Answer from the drawing. Dimensions are ordinates in mm from the lowest x, y and z of the part. Coordinates: 2 decimals unless noted, no trailing zeros. Loops run counter-clockwise (first coordinate to the right, second up) from the corner with the lowest first, then second, coordinate; pieces in that order, holes last. Notation, with made-up numbers: (58.25, -23) - (70.25, -23) arc R14 ccw to (70.25, -16) - close; hole circle Ø4 at (40, -18). An arc over 180 degrees is marked (long way). Write each question's results on one line, items separated by ' | '. Start each with the question number.
1. A cutting plane is placed at B-B on z = 25. Determine the outline of the cut face in (x, y), then the cut area to 3 significant figures.
2. Find the intervals of material crossed by line 1 along Z through (x, y) = (3, 93.85); line 2 along Y through (x, z) = (7.5, 25); line 3 along Y through (x, z) = (5.25, 31), in increasing order. Write a range as [from, to].
3. A cutting plane is placed at C-C on x = 5.75. Determine the outline of the cut face in (y, z).
4. A cutting plane is placed at A-A on y = 93.85. Determine the outline of the cut face in (x, z).
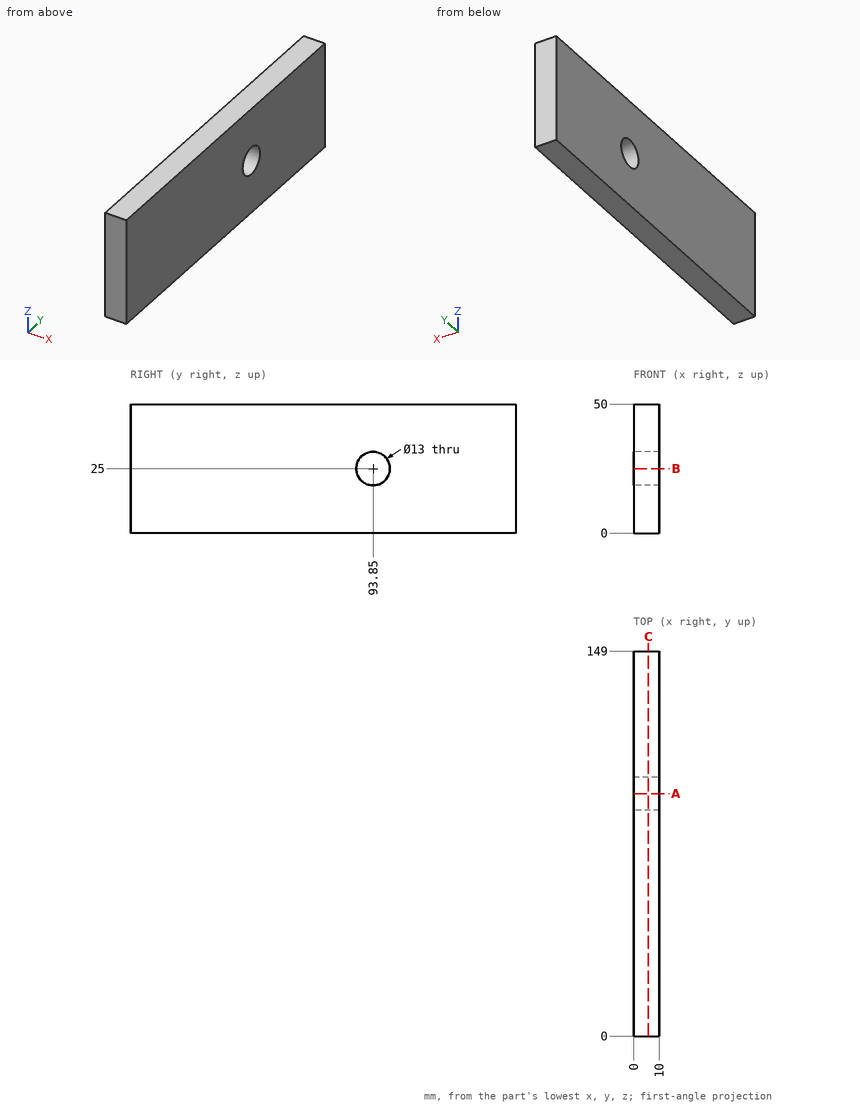
Values:
1) outline: (0, 0) - (10, 0) - (10, 87.35) - (0, 87.35) - close; (0, 100.35) - (10, 100.35) - (10, 149) - (0, 149) - close | area: 1,360 mm^2
2) line 1: [0, 18.5], [31.5, 50] | line 2: [0, 87.35], [100.35, 149] | line 3: [0, 91.35], [96.35, 149]
3) outline: (0, 0) - (149, 0) - (149, 50) - (0, 50) - close; hole circle Ø13 at (93.85, 25)
4) outline: (0, 0) - (10, 0) - (10, 18.5) - (0, 18.5) - close; (0, 31.5) - (10, 31.5) - (10, 50) - (0, 50) - close
